The model under review builds one solid part; all positions refer to its coordinate system, in mm. Face numbers are marked on the shaded views. A direction names the side the tool comes from. Give positions to 0.01 mm unless a question says otherwise; leave off trailing zeros. Loops run counter-clockwise (first coordinate to the right, second up) from the corner with the lowest first, then second, coordinate; pieces in that order, holes last. Notation, with made-up numbers: (79, -30) - (110, -30) arc R25 ccw to (110, 1) - close; hole circle Ø10 at (-17.5, 69.25). An arc over 180 degrees is marked (long way). Answer as a JSON object with one key per item and string values.
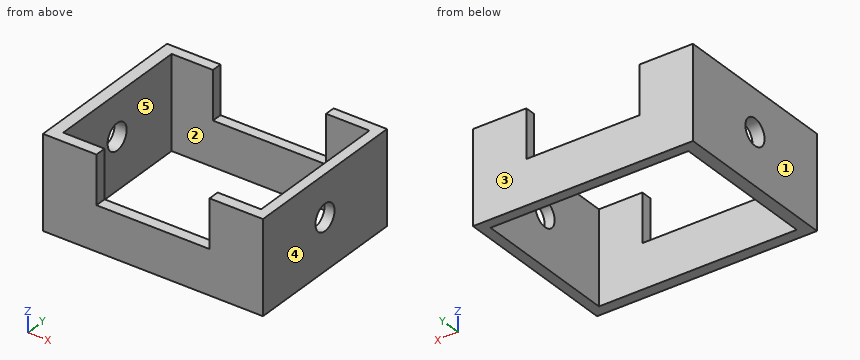
from build123d import *

# Parameters (mm, degrees)
F0_W     = 213.741392
F0_H     = 164.952264
F1_DEPTH = 89.916
F2_W     = 192.237719
F2_H     = 144.178293
F3_DEPTH = 137.668
F4_W     = 109.89108
F4_H     = 46.888998
F5_DEPTH = 190.246
F6_R     = 12.708744
F7_DEPTH = 299.212


with BuildPart() as f1:
    # F0 (on Top) → F1 (new body)
    with BuildSketch(Plane.XY):
        Rectangle(F0_W, F0_H)
    extrude(amount=F1_DEPTH)

    # F2 (on face) → F3 (cut)
    with BuildSketch(Plane.XY.offset(89.916)):
        with Locations((1.00965, 0.403863)):
            Rectangle(F2_W, F2_H)
    extrude(amount=-F3_DEPTH, mode=Mode.SUBTRACT)

    # F4 (on face) → F5 (cut)
    with BuildSketch(Plane.XZ.offset(82.476132)):
        with Locations((0, 66.471501)):
            Rectangle(F4_W, F4_H)
    extrude(amount=-F5_DEPTH, mode=Mode.SUBTRACT)

    # F6 (on face) → F7 (cut)
    with BuildSketch(Plane.YZ.offset(106.870696)):
        with Locations((0, 49.824677)):
            Circle(F6_R)
    extrude(amount=-F7_DEPTH, mode=Mode.SUBTRACT)


solid = f1.part
Q1. Consider section A-A, the plane z = 78. State the section outline as (x, y) points.
Results:
{"outline": "(-106.87, -82.48) - (-54.95, -82.48) - (-54.95, -71.69) - (-95.11, -71.69) - (-95.11, 72.49) - (-54.95, 72.49) - (-54.95, 82.48) - (-106.87, 82.48) - close; (54.95, -82.48) - (106.87, -82.48) - (106.87, 82.48) - (54.95, 82.48) - (54.95, 72.49) - (97.13, 72.49) - (97.13, -71.69) - (54.95, -71.69) - close"}
Q2. Consider section D-D, the plane z = 29.5. State the section outline as (x, y) points, plus the area to 3 significant figures.
Results:
{"outline": "(-106.87, -82.48) - (106.87, -82.48) - (106.87, 82.48) - (-106.87, 82.48) - close; hole (-95.11, -71.69) - (97.13, -71.69) - (97.13, 72.49) - (-95.11, 72.49) - close", "area": "7,540 mm^2"}
Q3. For the marked faces 1 and 2, list the 3-axis set-ups (+Z, -Z, +X, -X, +Y, -Y) from which the entire face can be reached by the end or side of a thin tool; tool diameter is ignored.
Results:
{"face 1": "+Z, -Z, -X, +Y, -Y", "face 2": "+Z, -Z"}
Q4. Clearance check with a flat-ended pin moving along its axis: pin 1 Ø8.5 at (x, y) = (-22, -77) entering from +Z. State where the tip first meets the part, or that it passes through.
Results:
{"pin 1": "stops at z = 43.03"}
Q5. Consider section C-C, the plane y = 62.5. State the section outline as (x, z) points.
Results:
{"outline": "(-106.87, 0) - (-95.11, 0) - (-95.11, 89.92) - (-106.87, 89.92) - close; (97.13, 0) - (106.87, 0) - (106.87, 89.92) - (97.13, 89.92) - close"}
Q6. Consider section B-B, the plane x = 51.5. State the section outline as (y, z) points.
Results:
{"outline": "(-82.48, 0) - (-71.69, 0) - (-71.69, 43.03) - (-82.48, 43.03) - close; (72.49, 0) - (82.48, 0) - (82.48, 43.03) - (72.49, 43.03) - close"}
Q7. To check wall thickness, follow probe 1 along Y at (x, z) = (-57, 33.5); probe 2 along X at (y, z) = (31, 7); probe 3 along Z at (x, y) = (-102.75, 0). State the ranges of each line that lie inside material, in increasing order. Write a range as [from, to].
Results:
{"probe 1": "y = [-82.48, -71.69], [72.49, 82.48]", "probe 2": "x = [-106.87, -95.11], [97.13, 106.87]", "probe 3": "z = [0, 37.12], [62.53, 89.92]"}
Q8. The part is to be moulded in two halves that separate along X. For the marked faces 3, 4 and 5, say which applies: +X half, -X half, draft (parallel to the pull), parting line (faces both ways), or undercut.
Results:
{"face 3": "draft", "face 4": "+X half", "face 5": "undercut"}
